Verification items for the finished model (mm, model axes). Give positions to 0.01 mm unless a question says otherwise; leave off trailing zeros. Write each loop counter-clockwise with the first axis right and the second up, starting at its lowest first coordinate (ties: lowest second). Pieces come first, ordered by that corner, then holes. Notation, with made-up numbers: (70, 85.25) -> (84, 85.25) arc R16 ccw to (84, 101.25) -> close; hole circle Ø10 at (49, 40). An arc over 180 degrees is marked (long way). Write item = value, one per line.
from build123d import *

# Parameters (mm, degrees)
BOSS_EXTRUDE1_DEPTH = 7.62
CUT_EXTRUDE1_START  = -8.62
SKETCH2_R           = 1.7399
CUT_EXTRUDE1_DEPTH  = 9.62


with BuildPart() as part:
    # Sketch1 → Boss-Extrude1 (new body)
    with BuildSketch(Plane.XY):
        with BuildLine():
            Line((0, 4.445), (86.36, 4.445))
            ThreePointArc((86.36, 4.445), (90.805, 0), (86.36, -4.445))
            Line((86.36, -4.445), (0, -4.445))
            ThreePointArc((0, -4.445), (-4.445, 0), (0, 4.445))
        make_face()
    extrude(amount=BOSS_EXTRUDE1_DEPTH)

    # Sketch2 → Cut-Extrude1 (cut)
    with BuildSketch(Plane.XY.offset(7.62).offset(CUT_EXTRUDE1_START)):
        Circle(SKETCH2_R)
    cut_extrude1 = extrude(amount=CUT_EXTRUDE1_DEPTH, mode=Mode.SUBTRACT)

    # Mirror1: Cut-Extrude1 across plane
    add(cut_extrude1.mirror(Plane(origin=(43.18, 0, 0), x_dir=(0, 0, 1), z_dir=(1, 0, 0))), mode=Mode.SUBTRACT)


solid = part.part
Item 1: Sectioned sample at A-A on y = 0. Record the cut outline in (x, z) (3 decimals), then the cut area to 3 significant figures.
Response values:
outline = (-4.445, 0) -> (-1.74, 0) -> (-1.74, 7.62) -> (-4.445, 7.62) -> close; (1.74, 0) -> (84.62, 0) -> (84.62, 7.62) -> (1.74, 7.62) -> close; (88.1, 0) -> (90.805, 0) -> (90.805, 7.62) -> (88.1, 7.62) -> close
area = 673 mm^2
Item 2: Mould release check, pull along X, two halves, no side actions. Record for faces 1 (the cylindrical face through (88.1, 0.08, 3.76)), 2 (the cylindrical face through (-4.444, -0.098, 3.757)), 3 (the flat face through (44, 0, 0)), 4 (the cylindrical face through (-1.38, -1.06, 3.76)): +X half, -X half, draft (parallel to the pull), parting line (faces both ways), or undercut.
Response values:
face_1 = undercut
face_2 = -X half
face_3 = draft
face_4 = undercut
Item 3: Go/stop test with flat-tipped pins: P1, Ø3, axis at x = 0, y = 0, coming from the +Z side; P2, Ø4, axis at y = 2.5, z = 2.5, coming from the +X side. Record where each tip stops, or that it passes through.
Response values:
P1 = through
P2 = 90.78
Item 4: Material ranges on line 1 (X direction, y = -0.5, z = 1.75); line 2 (Y direction, x = 86.36, z = 3) (3 decimals); line 3 (X direction, y = -1, z = 3.25), recorded low to high.
Response values:
line_1 = -4.42 to -1.67, 1.67 to 84.69, 88.03 to 90.78
line_2 = -4.445 to -1.74, 1.74 to 4.445
line_3 = -4.33 to -1.42, 1.42 to 84.94, 87.78 to 90.69
Item 5: Sectioned sample at B-B on z = 4.5. Record the cut outline in (x, y) (3 decimals).
Response values:
outline = (0, -4.445) -> (86.36, -4.445) arc R4.445 ccw to (86.36, 4.445) -> (0, 4.445) arc R4.445 ccw to start; hole circle Ø3.48 at (0, 0); hole circle Ø3.48 at (86.36, 0)
